```python
from build123d import *

# Parameters (mm, degrees)
ESBO_O1_R                = 1.7
RESSALTO_EXTRUS_O1_DEPTH = 3
FILETE1_R                = 20


with BuildPart() as part:
    # Esboço1 → Ressalto-extrusão1 (new body)
    with BuildSketch(Plane.XY):
        with BuildLine():
            Line((5.590169944, -5), (54.409830056, -5))
            ThreePointArc((54.409830056, -5), (67.5, 0), (54.409830056, 5))
            Line((54.409830056, 5), (5.590169944, 5))
            ThreePointArc((5.590169944, 5), (-7.5, 0), (5.590169944, -5))
        make_face()
        Circle(ESBO_O1_R, mode=Mode.SUBTRACT)
        with Locations((60, 0)):
            Circle(ESBO_O1_R, mode=Mode.SUBTRACT)
        with BuildLine():
            Line((30.901387819, -1.5), (36.5, -1.5))
            Line((36.5, -1.5), (36.5, 1.5))
            Line((36.5, 1.5), (30.901387819, 1.5))
            ThreePointArc((30.901387819, 1.5), (30, 1.75), (29.098612181, 1.5))
            Line((29.098612181, 1.5), (23.5, 1.5))
            Line((23.5, 1.5), (23.5, -1.5))
            Line((23.5, -1.5), (29.098612181, -1.5))
            ThreePointArc((29.098612181, -1.5), (30, -1.75), (30.901387819, -1.5))
        make_face(mode=Mode.SUBTRACT)
    extrude(amount=RESSALTO_EXTRUS_O1_DEPTH)

    # Filete1
    filete1_edges = [part.edges().sort_by_distance(p)[0] for p in [
        (54.409830056, -5, 1.5),
        (5.590169944, -5, 1.5),
        (5.590169944, 5, 1.5),
        (54.409830056, 5, 1.5),
    ]]
    fillet(filete1_edges, radius=FILETE1_R)


solid = part.part
```
Build history of the part. All positions in model axes, mm. A direction names the side the tool comes from. Coordinates: 2 decimals unless noted, no trailing zeros. Order: outer loops, then holes, each group sorted by start corner. A loop starts at its lowest first (then second) coordinate and runs counter-clockwise, first axis right, second up. Notation, with made-up numbers: (-22, 41) -> (-5, 41) arc R19 cw to (-5, 55) -> close; hole circle Ø10 at (75.25, 15). An arc over 180 degrees is marked (long way). Answer in a Markdown table with one row per item. Add a question column.
Q1. Band-saw the part on A-A, the plane x = 60. List the corners of the cut face in (y, z), then the cut area to 3 significant figures.
Q2. Band-saw the part on C-C, the plane z = 2.15. List the corners of the cut face in (x, y).
Q3. Mould opens along X. For faces 1 (the face through (29, 2, 3)), 2 (the face through (-0.37, -1.66, 1.48)), 3 (the face through (58.3, 0.07, 1.48)) say: +X half, -X half, draft (parallel to the pull), parting line (faces both ways), or undercut.
Q4. Band-saw the part on D-D, the plane x = 17. List the corners of the cut face in (y, z), then the cut area to 3 significant figures.
Q5. Which spindle directions (+Z, -Z, +X, -X, +Y, -Y) get a long thin tool onto all of the face, cutting with end or side? Do faces 4 (the face through (26, 1.5, 1)), 5 (the face through (30, -5, 1)), 6 (the face through (29, 2, 0)), 7 (the face through (7.134, 5.473, 1.521)). Say none if no direction does.
Q6. Drop flat-ended pins along their axis: pin 1 (0.9 mm diameter, centred on x = 26.5, z = 1.5, fed in from +Y); pin 2 (0.9 mm diameter, centred on x = 27.5, z = 1, fed in from -Y). Give the stop position or say it passes through.
Q7. Band-saw the part on B-B, the plane y = 0. List the corners of the cut face in (x, z), then the cut area to 3 significant figures.
Q8. Wall check: line 1 along Y through (x, z) = (0, 1.55); line 2 along Y through (x, z) = (44, 1.3); line 3 along Y through (x, z) = (25.5, 0.2). Give the ranges that are in metal, low to high. Write a range as [from, to].
Answers follow:
| question | item | result |
|---|---|---|
| 1 | outline | (-7.5, 0) -> (-1.7, 0) -> (-1.7, 3) -> (-7.5, 3) -> close; (1.7, 0) -> (7.5, 0) -> (7.5, 3) -> (1.7, 3) -> close |
| 1 | area | 34.8 mm^2 |
| 2 | outline | (3.12, -6.82) arc R20 cw to (11.46, -5) -> (48.54, -5) arc R20 cw to (56.88, -6.82) arc R7.5 ccw (long way) to (56.88, 6.82) arc R20 cw to (48.54, 5) -> (11.46, 5) arc R20 cw to (3.12, 6.82) arc R7.5 ccw (long way) to start; hole circle Ø3.4 at (0, 0); hole (23.5, -1.5) -> (29.1, -1.5) arc R1.75 ccw to (30.9, -1.5) -> (36.5, -1.5) -> (36.5, 1.5) -> (30.9, 1.5) arc R1.75 ccw to (29.1, 1.5) -> (23.5, 1.5) -> close; hole circle Ø3.4 at (60, 0) |
| 3 | face 1 | draft |
| 3 | face 2 | undercut |
| 3 | face 3 | undercut |
| 4 | outline | (-5, 0) -> (5, 0) -> (5, 3) -> (-5, 3) -> close |
| 4 | area | 30.0 mm^2 |
| 5 | face 4 | +Z, -Z |
| 5 | face 5 | +Z, -Z, -Y |
| 5 | face 6 | -Z, +X, -X, +Y, -Y |
| 5 | face 7 | +Z, -Z, +Y |
| 6 | pin 1 | y = 5 |
| 6 | pin 2 | y = -5 |
| 7 | outline | (-7.5, 0) -> (-1.7, 0) -> (-1.7, 3) -> (-7.5, 3) -> close; (1.7, 0) -> (23.5, 0) -> (23.5, 3) -> (1.7, 3) -> close; (36.5, 0) -> (58.3, 0) -> (58.3, 3) -> (36.5, 3) -> close; (61.7, 0) -> (67.5, 0) -> (67.5, 3) -> (61.7, 3) -> close |
| 7 | area | 166 mm^2 |
| 8 | line 1 | [-7.5, -1.7], [1.7, 7.5] |
| 8 | line 2 | [-5, 5] |
| 8 | line 3 | [-5, -1.5], [1.5, 5] |
